```python
from build123d import *

# Parameters (mm, degrees)
ESQUISSE1_W             = 26.25
ESQUISSE1_H             = 55
BOSS_EXTRU_1_DEPTH      = 5
BOSS_EXTRU_2_DEPTH      = 5
BOSS_EXTRU_3_DEPTH      = 5
ENL_V_MAT_EXTRU_1_DEPTH = 5
ESQUISSE5_W             = 50
ESQUISSE5_H             = 5
BOSS_EXTRU_4_DEPTH      = 36.25
BOSS_EXTRU_5_DEPTH      = 5
BOSS_EXTRU_6_DEPTH      = 5
BOSS_EXTRU_7_DEPTH      = 5
D_GAGEMENT_M301_D       = 34.65
D_GAGEMENT_M301_DEPTH   = 5
CONG_1_R                = 1.6
ESQUISSE11_W            = 20.033305553
ESQUISSE11_H            = 6.190231364
ESQUISSE11_W_2          = 5
ESQUISSE11_H_2          = 2.95
BOSS_EXTRU_8_DEPTH      = 5
ESQUISSE12_W            = 3.1
ESQUISSE12_H            = 4
ESQUISSE12_H_2          = 3
ESQUISSE12_W_2          = 1.23
ESQUISSE12_W_3          = 1.22
ESQUISSE12_W_4          = 4
ESQUISSE12_H_3          = 3.1
ESQUISSE12_W_5          = 3
ESQUISSE12_H_4          = 1.23
ESQUISSE12_H_5          = 1.22
ENL_V_MAT_EXTRU_2_DEPTH = 6


with BuildPart() as part:
    # Esquisse1 → Boss.-Extru.1 (new body)
    with BuildSketch(Plane(origin=(0, 5, 0), x_dir=(1, 0, 0), z_dir=(0, 1, 0))):
        with Locations((18.125, 0)):
            Rectangle(ESQUISSE1_W, ESQUISSE1_H)
    extrude(amount=-BOSS_EXTRU_1_DEPTH)

    # Esquisse2 → Boss.-Extru.2 (add)
    with BuildSketch(Plane(origin=(31.25, 0, 0), x_dir=(0, 0, -1), z_dir=(1, 0, 0))):
        Polygon((27.5, 5), (27.5, 0), (15.45, 0), (12.5, 2.95), (12.5, 5), align=None)
    extrude(amount=BOSS_EXTRU_2_DEPTH)

    # Esquisse3 → Boss.-Extru.3 (add)
    with BuildSketch(Plane(origin=(31.25, 0, 0), x_dir=(0, 0, -1), z_dir=(1, 0, 0))):
        Polygon((-15.45, 0), (-27.5, 0), (-27.5, 5), (-12.5, 5), (-12.5, 2.95), align=None)
    extrude(amount=BOSS_EXTRU_3_DEPTH)

    # Esquisse4 → Enlèv. mat.-Extru.1 (cut)
    with BuildSketch(Plane(origin=(0, 0, -27.5), x_dir=(-1, 0, 0), z_dir=(0, 0, -1))):
        Polygon((-5, 0), (-5, 2.95), (-7.95, 0), align=None)
    extrude(amount=-ENL_V_MAT_EXTRU_1_DEPTH, mode=Mode.SUBTRACT)

    # Esquisse5 → Boss.-Extru.4 (add)
    with BuildSketch(Plane.ZY.offset(-5)):
        with Locations((2.5, 2.5)):
            Rectangle(ESQUISSE5_W, ESQUISSE5_H)
    extrude(amount=BOSS_EXTRU_4_DEPTH)

    # Esquisse6 → Boss.-Extru.5 (add)
    with BuildSketch(Plane.ZY.offset(31.25)):
        Polygon((27.5, 5), (27.5, 0), (15.45, 0), (12.5, 2.95), (12.5, 5), align=None)
    extrude(amount=BOSS_EXTRU_5_DEPTH)

    # Esquisse7 → Boss.-Extru.6 (add)
    with BuildSketch(Plane.ZY.offset(31.25)):
        Polygon((-22.5, 5), (-12.5, 5), (-12.5, 2.95), (-15.45, 0), (-22.5, 0), align=None)
    extrude(amount=BOSS_EXTRU_6_DEPTH)

    # Esquisse8 → Boss.-Extru.7 (add)
    with BuildSketch(Plane(origin=(0, 0, -22.5), x_dir=(-1, 0, 0), z_dir=(0, 0, -1))):
        Polygon((5, 2.95), (5, 5), (36.25, 5), (36.25, 0), (7.95, 0), align=None)
    extrude(amount=BOSS_EXTRU_7_DEPTH)

    # Dégagement M301
    with Locations(Plane(origin=(0, 5, 0), x_dir=(1, 0, 0), z_dir=(0, 1, 0))):
        with Locations((0, -2.5)):
            Hole(D_GAGEMENT_M301_D / 2, depth=D_GAGEMENT_M301_DEPTH)

    # Congé1
    cong_1_edges = [part.edges().sort_by_distance(p)[0] for p in [
        (-5, 2.95, -25),
        (33.75, 2.95, -12.5),
        (33.75, 2.95, 12.5),
        (5, 2.95, -25),
        (-33.75, 2.95, 12.5),
        (-33.75, 2.95, -12.5),
    ]]
    fillet(cong_1_edges, radius=CONG_1_R)

    # Esquisse11 → Boss.-Extru.8 (add)
    with BuildSketch(Plane.XZ):
        with Locations((0.06715792, -24.404884318)):
            Rectangle(ESQUISSE11_W, ESQUISSE11_H)
        with Locations((-33.75, -13.975)):
            Rectangle(ESQUISSE11_W_2, ESQUISSE11_H_2)
        with Locations((-33.75, 13.975)):
            Rectangle(ESQUISSE11_W_2, ESQUISSE11_H_2)
        with Locations((33.75, 13.975)):
            Rectangle(ESQUISSE11_W_2, ESQUISSE11_H_2)
        with Locations((33.75, -13.975)):
            Rectangle(ESQUISSE11_W_2, ESQUISSE11_H_2)
    extrude(amount=-BOSS_EXTRU_8_DEPTH)

    # Esquisse12 → Enlèv. mat.-Extru.2 (cut, through all)
    with BuildSketch(Plane.XZ):
        with Locations((0, -25.5)):
            Rectangle(ESQUISSE12_W, ESQUISSE12_H)
        with Locations((0, -22)):
            Rectangle(ESQUISSE12_W, ESQUISSE12_H_2)
        with Locations((2.165, -22)):
            Rectangle(ESQUISSE12_W_2, ESQUISSE12_H_2)
        with Locations((0, -19)):
            Rectangle(ESQUISSE12_W, ESQUISSE12_H_2)
        with Locations((-2.16, -22)):
            Rectangle(ESQUISSE12_W_3, ESQUISSE12_H_2)
        with Locations((29.25, 0)):
            Rectangle(ESQUISSE12_W_4, ESQUISSE12_H_3)
        with Locations((25.75, 0)):
            Rectangle(ESQUISSE12_W_5, ESQUISSE12_H_3)
        with Locations((25.75, -2.165)):
            Rectangle(ESQUISSE12_W_5, ESQUISSE12_H_4)
        with Locations((22.75, 0)):
            Rectangle(ESQUISSE12_W_5, ESQUISSE12_H_3)
        with Locations((25.75, 2.16)):
            Rectangle(ESQUISSE12_W_5, ESQUISSE12_H_5)
        with Locations((-22.75, 0)):
            Rectangle(ESQUISSE12_W_5, ESQUISSE12_H_3)
        with Locations((-25.75, 0)):
            Rectangle(ESQUISSE12_W_5, ESQUISSE12_H_3)
        with Locations((-25.75, -2.165)):
            Rectangle(ESQUISSE12_W_5, ESQUISSE12_H_4)
        with Locations((-29.25, 0)):
            Rectangle(ESQUISSE12_W_4, ESQUISSE12_H_3)
        with Locations((-25.75, 2.16)):
            Rectangle(ESQUISSE12_W_5, ESQUISSE12_H_5)
    extrude(amount=-ENL_V_MAT_EXTRU_2_DEPTH, mode=Mode.SUBTRACT)


solid = part.part
```
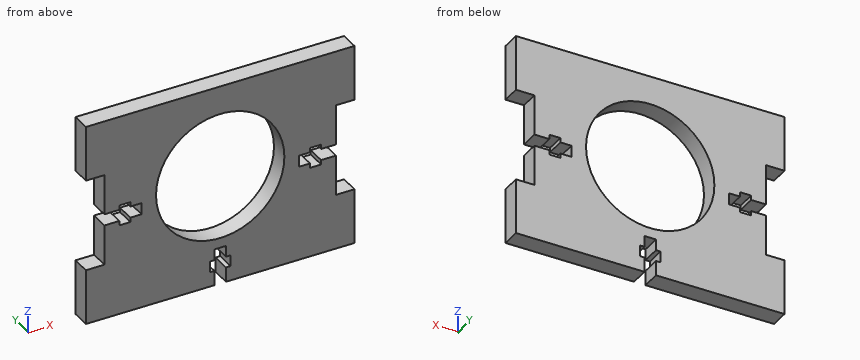
Build history of the part. All positions in model axes, mm. Coordinates: 2 decimals unless noted, no trailing zeros. Order: outer loops, then holes, each group sorted by start corner. A loop starts at its lowest first (then second) coordinate and runs counter-clockwise, first axis right, second up. Notation, with made-up numbers: (48, -31.75) -> (54, -31.75) arc R23 cw to (54, -19.75) -> close; hole circle Ø1 at (9, 87). An arc over 180 degrees is marked (long way). Answer in a Markdown table with one row per item. Add a question column.
Q1. Band-saw the part on A-A, the plane z = -21.5. List the corners of the cut face in (x, y).
Q2. Drop flat-ended pins along their axis: pin 1 (1.5 mm diameter, centred on y = 1, z = -9, fed in from +X); pin 2 (0.6 mm diameter, centred on y = 3, z = -2.5, fed in from -X). Give the stop position or say it passes through.
Q3. Wall check: line 1 along Z through (x, y) = (0, 3.4) (3 decimals); line 2 along Z through (x, y) = (24, 3.7); line 3 along X through (y, z) = (2.35, -7.5). Give the ranges that are in metal, low to high. Write a range as [from, to].
Q4. Band-saw the part on B-B, the plane x = 26.5. List the corners of the cut face in (y, z), then the cut area to 3 significant figures.
Answers follow:
| question | item | result |
|---|---|---|
| 1 | outline | (-36.25, 0) -> (-2.77, 0) -> (-2.77, 5) -> (-36.25, 5) -> close; (2.78, 0) -> (36.25, 0) -> (36.25, 5) -> (2.78, 5) -> close |
| 2 | pin 1 | x = 31.25 |
| 2 | pin 2 | x = -31.25 |
| 3 | line 1 | [-17.5, -14.825], [19.825, 27.5] |
| 3 | line 2 | [-27.5, -1.55], [1.55, 27.5] |
| 3 | line 3 | [-31.25, -14.15], [14.15, 31.25] |
| 4 | outline | (0, -27.5) -> (5, -27.5) -> (5, -2.78) -> (0, -2.78) -> close; (0, 2.77) -> (5, 2.77) -> (5, 27.5) -> (0, 27.5) -> close |
| 4 | area | 247 mm^2 |
